Here's how the part is built. I have some questions about the finished solid (model axes, mm). A direction names the side the tool comes from. Give positions to 0.01 mm unless a question says otherwise; leave off trailing zeros. Loops run counter-clockwise (first coordinate to the right, second up) from the corner with the lowest first, then second, coordinate; pieces in that order, holes last. Notation, with made-up numbers: (-1, -24) - (46, -24) arc R7 cw to (46, -14) - close; hole circle Ø11 at (32, 81.5). An arc over 180 degrees is marked (long way). One line per item, written item: value. Start each with the question number.
```python
from build123d import *

# Parameters (mm, degrees)
SKETCH1_W               = 3.5
SKETCH1_H               = 30
SKETCH1_W_2             = 23.825
SKETCH1_H_2             = 3
BOSS_EXTRUDE1_DEPTH     = 50
BOSS_EXTRUDE2_DEPTH     = 3.5
CUT_EXTRUDE1_START      = -28.325
SKETCH3_R               = 1.5
CUT_EXTRUDE1_DEPTH      = 29.325
SKETCH4_R               = 2.5
CUT_EXTRUDE2_DEPTH      = 1
CUT_EXTRUDE2_DEPTH_BACK = 3.15
SKETCH5_R               = 2.9
CUT_EXTRUDE3_DEPTH      = 7.15
CUT_EXTRUDE4_DEPTH      = 7.15
SKETCH7_R               = 2.5
SKETCH7_R_2             = 1.5
BOSS_EXTRUDE3_DEPTH     = 0.65
SKETCH9_R               = 6.5
CUT_EXTRUDE5_DEPTH      = 0.4
SKETCH12_R              = 4.4
BOSS_EXTRUDE4_DEPTH     = 1.13
SKETCH13_R              = 2.5
SKETCH13_R_2            = 1.5
BOSS_EXTRUDE5_DEPTH     = 2.5
SKETCH14_R              = 2.65
CUT_EXTRUDE7_DEPTH      = 5.05
SKETCH10_R              = 4.4
CUT_EXTRUDE8_DEPTH      = 10
CUT_EXTRUDE8_DEPTH_BACK = 10


with BuildPart() as part:
    # Sketch1 → Boss-Extrude1 (new body)
    with BuildSketch(Plane.XY):
        with Locations((-25.575, -15)):
            Rectangle(SKETCH1_W, SKETCH1_H)
        with Locations((-11.9125, -28.5)):
            Rectangle(SKETCH1_W_2, SKETCH1_H_2)
    boss_extrude1 = extrude(amount=BOSS_EXTRUDE1_DEPTH)

    # Sketch2 → Boss-Extrude2 (add)
    with BuildSketch(Plane(origin=(-23.825, 0, 0), x_dir=(0, 0, -1), z_dir=(1, 0, 0))):
        with BuildLine():
            Line((8, 0), (6.5, 0))
            ThreePointArc((6.5, 0), (4.596194078, -4.596194078), (0, -6.5))
            Line((0, -6.5), (0, -27))
            Line((0, -27), (0, -30))
            Line((0, -30), (8, -30))
            Line((8, -30), (8, 0))
        make_face()
        with BuildLine():
            Line((6.5, 0), (1.5, 0))
            ThreePointArc((1.5, 0), (1.060660172, -1.060660172), (0, -1.5))
            Line((0, -1.5), (0, -6.5))
            ThreePointArc((0, -6.5), (4.596194078, -4.596194078), (6.5, 0))
        make_face()
        with BuildLine():
            ThreePointArc((-1.5, 0), (0, 1.5), (1.5, 0))
            Line((1.5, 0), (6.5, 0))
            ThreePointArc((6.5, 0), (0, 6.5), (-6.5, 0))
            Line((-6.5, 0), (-1.5, 0))
        make_face()
    boss_extrude2 = extrude(amount=-BOSS_EXTRUDE2_DEPTH)

    # Sketch3 → Cut-Extrude1 (cut)
    with BuildSketch(Plane.ZY.offset(27.325).offset(CUT_EXTRUDE1_START)):
        Circle(SKETCH3_R)
    cut_extrude1 = extrude(amount=CUT_EXTRUDE1_DEPTH, mode=Mode.SUBTRACT)

    # Mirror1: Boss-Extrude1, Boss-Extrude2, Cut-Extrude1 across plane
    add(boss_extrude1.mirror(Plane(origin=(0, 0, 50), x_dir=(0, 0, 1), z_dir=(-1, 0, 0))))
    add(boss_extrude2.mirror(Plane(origin=(0, 0, 50), x_dir=(0, 0, 1), z_dir=(-1, 0, 0))))
    add(cut_extrude1.mirror(Plane(origin=(0, 0, 50), x_dir=(0, 0, 1), z_dir=(-1, 0, 0))), mode=Mode.SUBTRACT)

    # Sketch4 → Cut-Extrude2 (cut, two sides)
    with BuildSketch(Plane.ZY.offset(27.325)) as cut_extrude2_sk:
        Circle(SKETCH4_R)
    extrude(amount=CUT_EXTRUDE2_DEPTH, mode=Mode.SUBTRACT)
    extrude(cut_extrude2_sk.sketch, amount=-CUT_EXTRUDE2_DEPTH_BACK, mode=Mode.SUBTRACT)

    # Sketch5 → Cut-Extrude3 (cut)
    with BuildSketch(Plane(origin=(27.325, 0, 0), x_dir=(0, 0, -1), z_dir=(1, 0, 0))):
        Circle(SKETCH5_R)
    extrude(amount=-CUT_EXTRUDE3_DEPTH, mode=Mode.SUBTRACT)

    # Sketch6 → Cut-Extrude4 (cut)
    with BuildSketch(Plane.ZY.offset(27.325)):
        Polygon((50, 0), (50, -25), (35, -5), (6.5, -5), (6.5, 0), align=None)
    cut_extrude4 = extrude(amount=-CUT_EXTRUDE4_DEPTH, mode=Mode.SUBTRACT)

    # Mirror2: Cut-Extrude4 across plane
    add(cut_extrude4.mirror(Plane(origin=(0, 0, 0), x_dir=(0, 0, 1), z_dir=(1, 0, 0))), mode=Mode.SUBTRACT)

    # Sketch7 → Boss-Extrude3 (add)
    with BuildSketch(Plane.ZY.offset(24.175)):
        Circle(SKETCH7_R)
        Circle(SKETCH7_R_2, mode=Mode.SUBTRACT)
    extrude(amount=BOSS_EXTRUDE3_DEPTH)

    # Sketch9 → Cut-Extrude5 (cut)
    with BuildSketch(Plane(origin=(27.325, 0, 0), x_dir=(0, 0, -1), z_dir=(1, 0, 0))):
        Circle(SKETCH9_R)
        Polygon((8, 0), (-6.5, 0), (-6.5, -3.791432832), (-52.61721684, -3.791432832), (-52.61721684, -30), (-6.5, -30), (8, -30), align=None)
    extrude(amount=-CUT_EXTRUDE5_DEPTH, mode=Mode.SUBTRACT)

    # Sketch12 → Boss-Extrude4 (add)
    with BuildSketch(Plane(origin=(26.925, 0, 0), x_dir=(0, 0, -1), z_dir=(1, 0, 0))):
        with BuildLine():
            Line((8, 0), (6.5, 0))
            ThreePointArc((6.5, 0), (0, 6.5), (-6.5, 0))
            Line((-6.5, 0), (-6.5, -5))
            Line((-6.5, -5), (-35, -5))
            Line((-35, -5), (-50, -25))
            Line((-50, -25), (-50, -30))
            Line((-50, -30), (8, -30))
            Line((8, -30), (8, 0))
        make_face()
        Circle(SKETCH12_R, mode=Mode.SUBTRACT)
    extrude(amount=BOSS_EXTRUDE4_DEPTH)

    # Sketch13 → Boss-Extrude5 (add)
    with BuildSketch(Plane.ZY.offset(27.325)):
        Circle(SKETCH13_R)
        Circle(SKETCH13_R_2, mode=Mode.SUBTRACT)
    extrude(amount=-BOSS_EXTRUDE5_DEPTH)

    # Sketch14 → Cut-Extrude7 (cut)
    with BuildSketch(Plane.ZY.offset(27.325)):
        Circle(SKETCH14_R)
    extrude(amount=-CUT_EXTRUDE7_DEPTH, mode=Mode.SUBTRACT)

    # Sketch10 → Cut-Extrude8 (cut, two sides)
    with BuildSketch(Plane(origin=(26.925, 0, 0), x_dir=(0, 0, -1), z_dir=(1, 0, 0))) as cut_extrude8_sk:
        Circle(SKETCH10_R)
    extrude(amount=CUT_EXTRUDE8_DEPTH, mode=Mode.SUBTRACT)
    extrude(cut_extrude8_sk.sketch, amount=-CUT_EXTRUDE8_DEPTH_BACK, mode=Mode.SUBTRACT)


solid = part.part
```
(1) If we section it at B-B on z = 10: List the corners of the cut face in (x, y) for me (3 decimals), plus the area to 3 significant figures.
(2) If we section it at C-C on y = -1: List the corners of the cut face in (x, z) for me (3 decimals).
(3) Will these pins go through, and if not, where does the flat tip stop? pin 1 (1.5 mm diameter, centred on x = -7.5, y = -28.5, fed in from -Z); pin 2 (4 mm diameter, centred on y = 0, z = 0, fed in from +X); pin 3 (4 mm diameter, centred on x = -26, y = -1.5, fed in from +Z); pin 4 (1.3 mm diameter, centred on x = 25.5, z = 19, fed in from +Y).
(4) If we section it at A-A on y = -7: List the corners of the cut face in (x, z) for me (3 decimals), plus the area to 3 significant figures.
(5) If we mould it in two halves opening along X, with no side actions, what happens to faces 6 (the face through (0, -28, 0)), 7 (the face through (-27.325, -16, 14)), 8 (the face through (-26, 0, -7))? For each: pulls with the +X half, pulls with the -X half, needs draft (parallel to the pull), parting line crosses it, or undercut.
(6) If we section it at D-D on x = 13: List the corners of the cut face in (y, z) for me, plus the area to 3 significant figures.
(7) For faces 1 (the face through (-25.6, 6.5, -0.1)), 2 (the face through (26, 0, -7)), 3 (the face through (26, -5, 21)), 4 (the face through (-25.6, -1.01, 2.45)), 5 (the face through (0, -27, 25)), which set-ups out of +Z, -Z, +X, -X, +Y, -Y let a thin tool reach every point of the face, with its end or its side?
(8) Please list where these lines run through material, in increasing order: probe 1 along X at (y, z) = (-17, 28) (3 decimals); probe 2 along Y at (x, z) = (-25, 0); probe 3 along Z at (x, y) = (25.5, -3.5). Write a range as from..to.
Found:
1. outline: (-27.325, -30) - (28.055, -30) - (28.055, -5) - (23.825, -5) - (23.825, -27) - (-23.825, -27) - (-23.825, -5) - (-27.325, -5) - close
1. area: 336 mm^2
2. outline: (-27.325, -8) - (-23.825, -8) - (-23.825, -2.454) - (-27.325, -2.454) - close; (-27.325, 2.454) - (-23.825, 2.454) - (-23.825, 6.5) - (-27.325, 6.5) - close; (23.825, -8) - (28.055, -8) - (28.055, -4.285) - (23.825, -4.285) - close; (23.825, 4.285) - (28.055, 4.285) - (28.055, 6.5) - (23.825, 6.5) - close
3. pin 1: z = 0
3. pin 2: through
3. pin 3: z = 6.5
3. pin 4: y = -5
4. outline: (-27.325, -8) - (-23.825, -8) - (-23.825, 36.5) - (-27.325, 36.5) - close; (23.825, -8) - (28.055, -8) - (28.055, 36.5) - (23.825, 36.5) - close
4. area: 344 mm^2
5. face 6: undercut
5. face 7: pulls with the -X half
5. face 8: needs draft
6. outline: (-30, 0) - (-27, 0) - (-27, 50) - (-30, 50) - close
6. area: 150 mm^2
7. face 1: +X, -X, +Y
7. face 2: -Z, +X, -X, +Y
7. face 3: +Z, +X, -X, +Y
7. face 4: +X, -X
7. face 5: +Z, -Z, +Y
8. probe 1: -27.325..-23.825, 23.825..28.055
8. probe 2: -30..-2.65, 2.65..6.5
8. probe 3: -8..-2.67, 2.67..6.5
